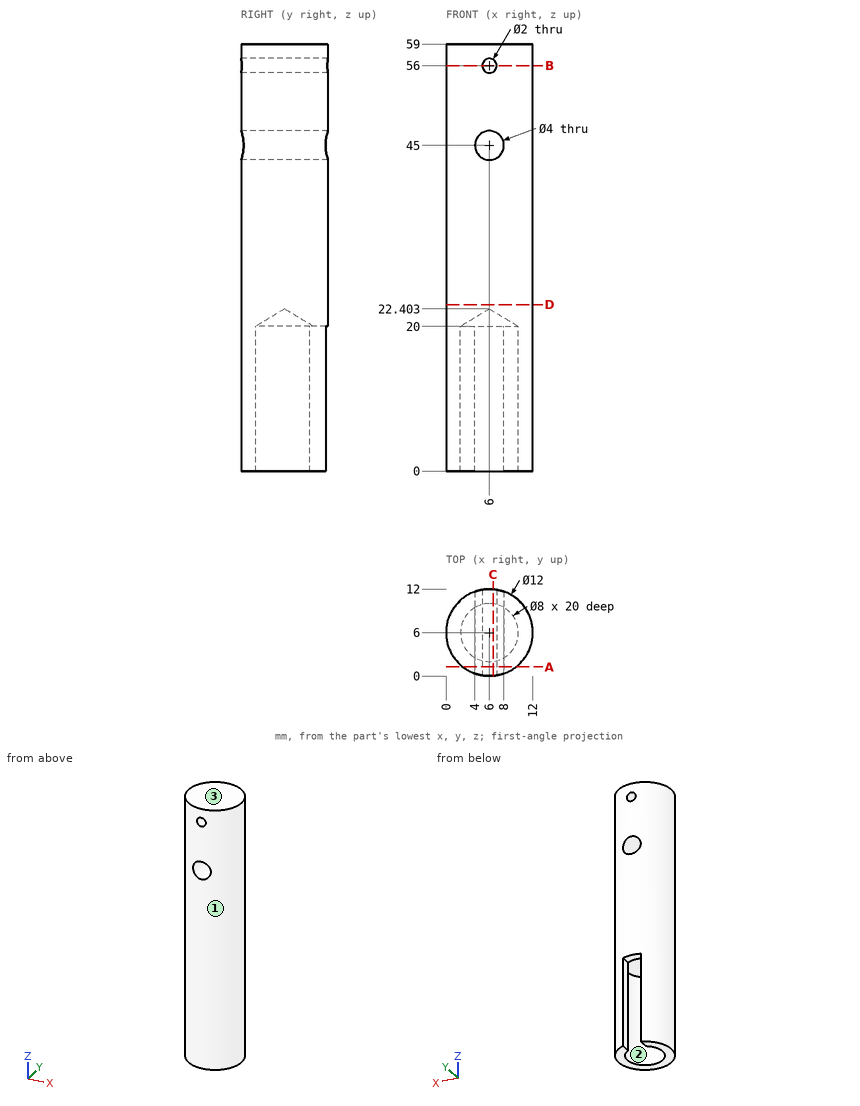
Geometry: see drawing. Coordinates: mm, zero at the bounding-box minimum. Give positions to 0.01 mm unless a question says otherwise; leave off trailing zeros. Order: outer loops, then holes, each group sorted by start corner. A loop starts at its lowest first (then second) coordinate and runs counter-clockwise, first axis right, second up. Notation, with made-up numbers: (65, 79.5) -> (82, 79.5) arc R12 ccw to (82, 86.5) -> close; hole circle Ø6 at (68, -37). An arc over 180 degrees is marked (long way). Write each question's results on one line, items separated by ' | '. Start each with the question number.
1) Section D-D (z = 23). Return loops of the section in (x, y).
2) Line query: line 1 (Z direction, x = 6.25, y = 4.5) (1 decimal); line 2 (Z direction, x = 6.25, y = 2.75) (1 decimal); line 3 (Y direction, x = 9.25, z = 15.5) (1 decimal). Output: solid intervals per line, ascending. Write a range as from..to.
3) Section A-A (y = 1.25). Return loops of the section in (x, z) (1 decimal), then the cut area to 3 significant figures.
4) Section B-B (z = 56). Return loops of the section in (x, y).
5) First-contact query: pin 1 (3 mm diameter, centred on x = 6, z = 45, fed in from +Y); pin 2 (3 mm diameter, centred on x = 2, z = 42, fed in from +Y) (1 decimal); pin 3 (2 mm diameter, centred on x = 6.5, y = 11.5, fed in from -Z); pin 4 (3 mm diameter, centred on y = 10.5, z = 10, fed in from -X) (1 decimal). Flat tips, straight axial feed; report the tip coordinate or a pass-through.
6) Draft query along Y for the marked faces 1, 2 and 3. Return one class per face: pulls with the +Y half, pulls with the -Y half, needs draft (parallel to the pull), parting line crosses it, or undercut.
7) Section C-C (x = 6.5). Count the separate pieces of the cut face and the enclosed holes in it.
Calculated:
1) outline: circle Ø12 at (6, 6)
2) line 1: 21.5..43, 47..55, 57..59 | line 2: 20.4..43, 47..55, 57..59 | line 3: 1..3.7, 8.3..11
3) outline: (2.3, 0) -> (9.7, 0) -> (9.7, 59) -> (2.3, 59) -> close; hole circle Ø4 at (6, 45); hole circle Ø2 at (6, 56) | area: 417 mm2
4) outline: (5, 0.08) -> (5, 11.92) arc R6 ccw to start; (7, 0.08) arc R6 ccw to (7, 11.92) -> close
5) pin 1: through | pin 2: y = 11.5 | pin 3: z = 20 | pin 4: x = 0.8
6) face 1: parting line crosses it | face 2: undercut | face 3: needs draft
7) separate pieces: 3 | enclosed holes: 0
